```python
from build123d import *

# Parameters (mm, degrees)
F0_R          = 9.525
F1_DEPTH      = 19.05
F2_R          = 3.175
F3_DEPTH      = 3.175
F4_R          = 3.175
F5_DEPTH      = 3.175
F6_R          = 3.175
F7_DEPTH      = 9.526
F7_DEPTH_BACK = 25.4
F8_SIZE       = 0.2286


with BuildPart() as f1:
    # F0 (on Top) → F1 (new body)
    with BuildSketch(Plane.XY):
        Circle(F0_R)
    extrude(amount=F1_DEPTH)

    # F2 (on face) → F3 (join)
    with BuildSketch(Plane.XY.offset(19.05)):
        Circle(F2_R)
    extrude(amount=F3_DEPTH)

    # F4 (on face) → F5 (join)
    with BuildSketch(Plane(origin=(0, 0, 0), x_dir=(1, 0, 0), z_dir=(0, 0, -1))):
        Circle(F4_R)
    extrude(amount=F5_DEPTH)

    # F6 (on Right) → F7 (cut, two sides)
    with BuildSketch(Plane.YZ) as f7_sk:
        with Locations((0, 9.525)):
            Circle(F6_R)
    extrude(amount=-F7_DEPTH, mode=Mode.SUBTRACT)
    extrude(f7_sk.sketch, amount=F7_DEPTH_BACK, mode=Mode.SUBTRACT)

    # F8
    f8_edges = [f1.edges().sort_by_distance(p)[0] for p in [
        (-3.175, 0, 22.225),
        (-9.525, 0, 19.05),
        (-3.175, 0, -3.175),
        (-9.525, 0, 0),
    ]]
    chamfer(f8_edges, length=F8_SIZE)


solid = f1.part
```
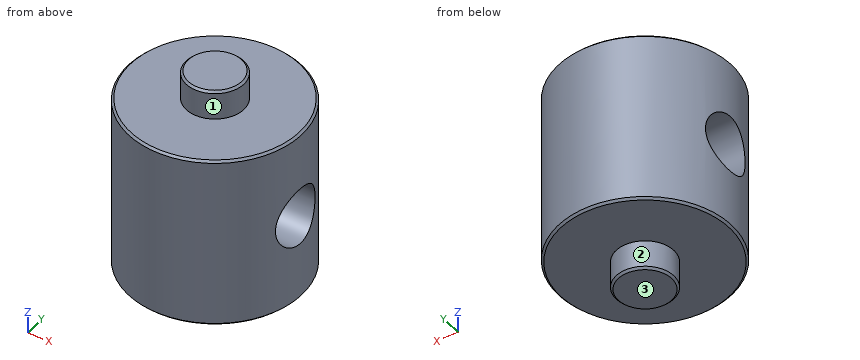
Read the model definition and answer for the solid it produces. Units are mm, in the model's axes. Face numbers are marked on the shaded views. A direction names the side the tool comes from. Coordinates: 2 decimals unless noted, no trailing zeros. Loops run counter-clockwise (first coordinate to the right, second up) from the corner with the lowest first, then second, coordinate; pieces in that order, holes last. Notation, with made-up numbers: (15.25, 89.5) -> (66.25, 89.5) arc R28 ccw to (66.25, 109.5) -> close; hole circle Ø11 at (63, 5.5). An arc over 180 degrees is marked (long way). Return JSON: item names as keys, results as strings.
Item 1: For the marked faces 1, 2 and 3, determine the directions among +Z, -Z, +X, -X, +Y, -Y from which every point of the face is accessible in a straight line to the end or side of a thin tool.
Answers:
{"face 1": "+Z", "face 2": "-Z", "face 3": "-Z, +X, -X, +Y, -Y"}
Item 2: Find section C-C (z = 8.75). Determine the outline of the cut face in (x, y) (3 decimals), plus the area to 3 significant figures.
Answers:
{"outline": "(-9.014, -3.079) arc R9.525 ccw to (9.014, -3.079) -> close; (-9.014, 3.079) -> (9.014, 3.079) arc R9.525 ccw to start", "area": "170 mm2"}
Item 3: Find section A-A (y = 0). Determine the outline of the cut face in (x, z) (3 decimals), plus the area to 3 significant figures.
Answers:
{"outline": "(-9.525, 0.229) -> (-9.296, 0) -> (-3.175, 0) -> (-3.175, -2.946) -> (-2.946, -3.175) -> (2.946, -3.175) -> (3.175, -2.946) -> (3.175, 0) -> (9.296, 0) -> (9.525, 0.229) -> (9.525, 6.35) -> (-9.525, 6.35) -> close; (-9.525, 12.7) -> (9.525, 12.7) -> (9.525, 18.821) -> (9.296, 19.05) -> (3.175, 19.05) -> (3.175, 21.996) -> (2.946, 22.225) -> (-2.946, 22.225) -> (-3.175, 21.996) -> (-3.175, 19.05) -> (-9.296, 19.05) -> (-9.525, 18.821) -> close", "area": "282 mm2"}
Item 4: Flat-ended cylindrical pins translate along their axes: P1, Ø5, axis at y = 6, z = 6.5, coming from the -X side; P2, Ø1.5, axis at x = 4, z = 16, coming from the -Y side; P3, Ø4, axis at x = 3.5, z = 9, coming from the +Y side; P4, Ø3, axis at y = -1.5, z = 9.5, coming from the -X side. Find the tip coordinate at first contact, or state that the pin passes through.
Answers:
{"P1": "stops at x = -8.86", "P2": "stops at y = -8.95", "P3": "stops at y = 9.41", "P4": "passes through"}
Item 5: Find section D-D (z = 16). Determine the outline of the cut face in (x, y) (3 decimals).
Answers:
{"outline": "circle Ø19.05 at (0, 0)"}
Item 6: Find section B-B (z = 19.5). Determine the outline of the cut face in (x, y) (3 decimals), plus the area to 3 significant figures.
Answers:
{"outline": "circle Ø6.35 at (0, 0)", "area": "31.7 mm2"}
Item 7: Find the intervals of material crossed by probe 1 along Z at (x, y) = (4.5, 0); probe 2 along Z at (x, y) = (2, 0) (3 decimals); probe 3 along Y at (x, z) = (-4, 8.5) (3 decimals), in increasing order.
Answers:
{"probe 1": "z = 0 to 6.35, 12.7 to 19.05", "probe 2": "z = -3.175 to 6.35, 12.7 to 22.225", "probe 3": "y = -8.644 to -3.005, 3.005 to 8.644"}
